```python
from build123d import *

# Parameters (mm, degrees)
SKETCH1_W             = 1075
SKETCH1_H             = 25
BOSS_EXTRUDE1_DEPTH   = 25
BOSS_EXTRUDE1_2_DEPTH = 25
SKETCH2_W             = 25
SKETCH2_H             = 25
BOSS_EXTRUDE2_DEPTH   = 285
BOSS_EXTRUDE3_REACH   = 918.164
SKETCH3_W             = 25
SKETCH3_H             = 25
SKETCH4_W             = 25
SKETCH4_H             = 25
BOSS_EXTRUDE4_DEPTH   = 75
SKETCH5_W             = 25
SKETCH5_H             = 25
BOSS_EXTRUDE5_DEPTH   = 190


with BuildPart() as part:
    # Sketch1 → Boss-Extrude1 (new body)
    with BuildSketch(Plane.XY):
        with Locations((0, -342.5)):
            Rectangle(SKETCH1_W, SKETCH1_H)
    extrude(amount=BOSS_EXTRUDE1_DEPTH)



with BuildPart() as body_2:
    # Sketch1 → Boss-Extrude1 2 (new body)
    with BuildSketch(Plane.XY):
        with Locations((0, 342.5)):
            Rectangle(SKETCH1_W, SKETCH1_H)
    extrude(amount=BOSS_EXTRUDE1_2_DEPTH)


with BuildPart() as part_1:
    add(part.part)

    add(body_2.part)  # Boss-Extrude2 merges body 2
    # Sketch2 → Boss-Extrude2 (add)
    with BuildSketch(Plane(origin=(0, 0, 0), x_dir=(-1, 0, 0), z_dir=(0, 0, -1))):
        with Locations((-525, 342.5)):
            Rectangle(SKETCH2_W, SKETCH2_H)
        with Locations((525, 342.5)):
            Rectangle(SKETCH2_W, SKETCH2_H)
        with Locations((525, -342.5)):
            Rectangle(SKETCH2_W, SKETCH2_H)
        with Locations((-525, -342.5)):
            Rectangle(SKETCH2_W, SKETCH2_H)
    extrude(amount=BOSS_EXTRUDE2_DEPTH)

    # Sketch3 → Boss-Extrude3 (add, up to next)
    with BuildSketch(Plane(origin=(0, -330, 0), x_dir=(1, 0, 0), z_dir=(0, 1, 0)), mode=Mode.PRIVATE) as boss_extrude3_sk1:
        with Locations((-525, 107.5)):
            Rectangle(SKETCH3_W, SKETCH3_H)
    boss_extrude3_tool1 = extrude(boss_extrude3_sk1.sketch, amount=BOSS_EXTRUDE3_REACH, mode=Mode.PRIVATE) - part_1.part
    # Sketch3 → Boss-Extrude3 (add, up to next)
    with BuildSketch(Plane(origin=(0, -330, 0), x_dir=(1, 0, 0), z_dir=(0, 1, 0)), mode=Mode.PRIVATE) as boss_extrude3_sk2:
        with Locations((525, 107.5)):
            Rectangle(SKETCH3_W, SKETCH3_H)
    boss_extrude3_tool2 = extrude(boss_extrude3_sk2.sketch, amount=BOSS_EXTRUDE3_REACH, mode=Mode.PRIVATE) - part_1.part
    add(boss_extrude3_tool1.solids().sort_by_distance((-525, -330, -107.5))[0])
    add(boss_extrude3_tool2.solids().sort_by_distance((525, -330, -107.5))[0])

    # Sketch4 → Boss-Extrude4 (add)
    with BuildSketch(Plane.XY.offset(25)):
        with Locations((-525, -342.5)):
            Rectangle(SKETCH4_W, SKETCH4_H)
        with Locations((525, -342.5)):
            Rectangle(SKETCH4_W, SKETCH4_H)
    extrude(amount=BOSS_EXTRUDE4_DEPTH)

    # Sketch5 → Boss-Extrude5 (add)
    with BuildSketch(Plane.XZ.offset(355)):
        with Locations((-525, -272.5)):
            Rectangle(SKETCH5_W, SKETCH5_H)
        with Locations((-525, 87.5)):
            Rectangle(SKETCH5_W, SKETCH5_H)
        with Locations((525, 87.5)):
            Rectangle(SKETCH5_W, SKETCH5_H)
        with Locations((525, -272.5)):
            Rectangle(SKETCH5_W, SKETCH5_H)
    extrude(amount=BOSS_EXTRUDE5_DEPTH)


solid = part_1.part
```
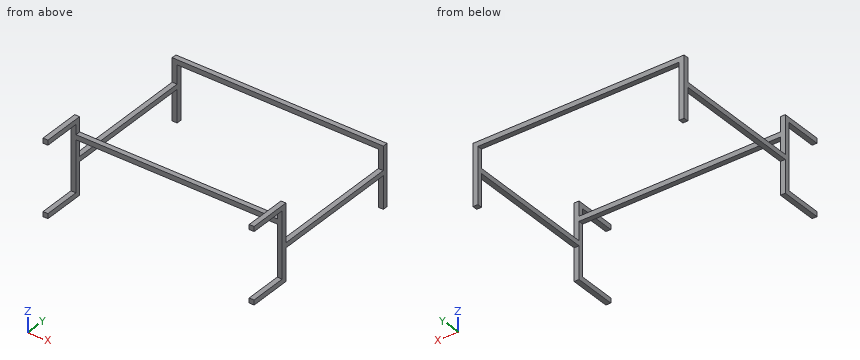
The model under review builds one solid part; all positions refer to its coordinate system, in mm. Coordinates: 2 decimals unless noted, no trailing zeros. Write each loop counter-clockwise with the first axis right and the second up, starting at its lowest first coordinate (ties: lowest second). Pieces come first, ordered by that corner, then holes. Notation, with made-up numbers: (44.5, -17.5) - (54.5, -17.5) arc R25 cw to (54.5, 21.5) - close; hole circle Ø1 at (23, 40). An arc over 180 degrees is marked (long way). Answer in a Markdown table with one row per item. Add a question column.
Q1. Consider section C-C on y = -412.5. Give the boundary of the cut face in (x, z), then the cut area to 3 significant figures.
Q2. To check wall thickness, follow line 1 along X through (y, z) = (-346.5, 84.5). State the ranges of the line that lie inside material, in increasing order. Write a range as from..to.
Q3. Consider section A-A on z = 57.5. Give the boundary of the cut face in (x, y), then the cut area to 3 significant figures.
Q4. Consider section D-D on z = -181. Give the boundary of the cut face in (x, y), then the cut area to 3 significant figures.
Q5. Clearance check with flat-ended pins moving along their axes: pin 1 (20 mm diameter, centred on x = -122, y = -342, fed in from -Z); pin 2 (20 mm diameter, centred on x = 520, y = -79, fed in from -Z); pin 3 (12.5 mm diameter, centred on x = -531, y = 25, fed in from +Z). State where each tip first meets the part, or that it passes through.
Q6. Consider section B-B on y = -110. Give the boundary of the cut face in (x, z), then the cut area to 3 significant figures.
Answers below:
| question | item | result |
|---|---|---|
| 1 | outline | (-537.5, -285) - (-512.5, -285) - (-512.5, -260) - (-537.5, -260) - close; (-537.5, 75) - (-512.5, 75) - (-512.5, 100) - (-537.5, 100) - close; (512.5, -285) - (537.5, -285) - (537.5, -260) - (512.5, -260) - close; (512.5, 75) - (537.5, 75) - (537.5, 100) - (512.5, 100) - close |
| 1 | area | 2,500 mm² |
| 2 | line 1 | -537.5..-512.5, 512.5..537.5 |
| 3 | outline | (-537.5, -355) - (-512.5, -355) - (-512.5, -330) - (-537.5, -330) - close; (512.5, -355) - (537.5, -355) - (537.5, -330) - (512.5, -330) - close |
| 3 | area | 1,250 mm² |
| 4 | outline | (-537.5, -355) - (-512.5, -355) - (-512.5, -330) - (-537.5, -330) - close; (-537.5, 330) - (-512.5, 330) - (-512.5, 355) - (-537.5, 355) - close; (512.5, -355) - (537.5, -355) - (537.5, -330) - (512.5, -330) - close; (512.5, 330) - (537.5, 330) - (537.5, 355) - (512.5, 355) - close |
| 4 | area | 2,500 mm² |
| 5 | pin 1 | z = 0 |
| 5 | pin 2 | z = -120 |
| 5 | pin 3 | z = -95 |
| 6 | outline | (-537.5, -120) - (-512.5, -120) - (-512.5, -95) - (-537.5, -95) - close; (512.5, -120) - (537.5, -120) - (537.5, -95) - (512.5, -95) - close |
| 6 | area | 1,250 mm² |
